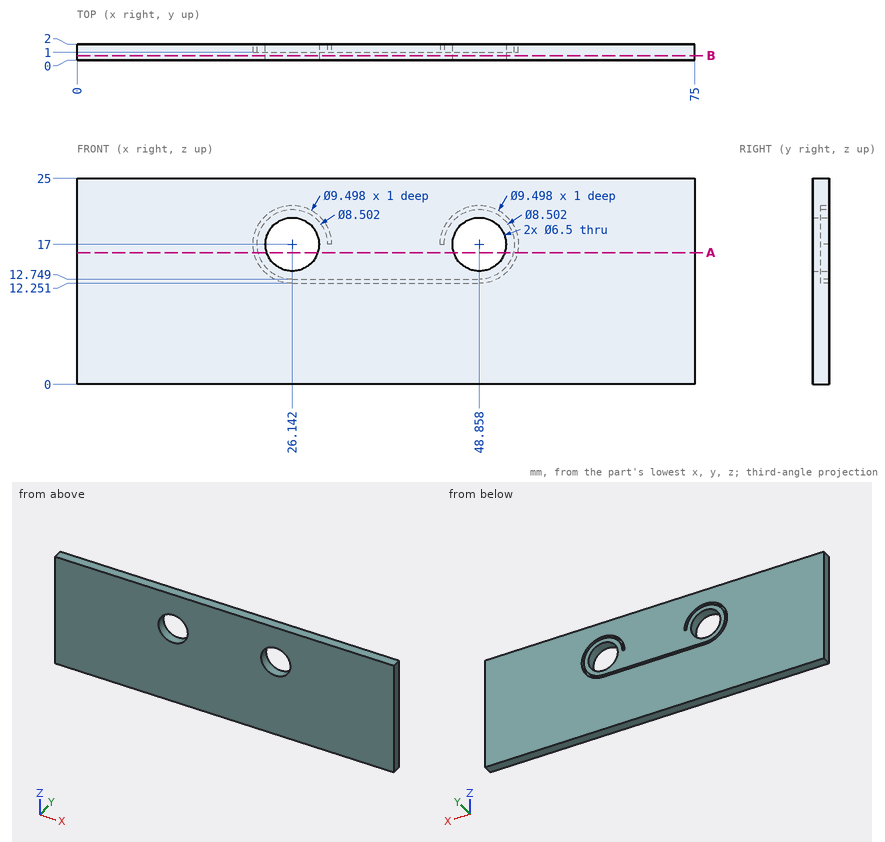
The drawing under review shows one solid part. Ordinate dimensions are in mm from its lowest x, y, z. Coordinates: 2 decimals unless noted, no trailing zeros. Loops run counter-clockwise (first coordinate to the right, second up) from the corner with the lowest first, then second, coordinate; pieces in that order, holes last. Notation, with made-up numbers: (86.25, 47) - (126.25, 47) arc R5 cw to (126.25, 55) - close; hole circle Ø7 at (76.25, 78). An arc over 180 degrees is marked (long way). Use CSV: the item, a comma, the result in double quotes. Start each with the question number.
1. Add section A-A on z = 16. Give the boundary of the cut face in (x, y), plus the area to 3 significant figures.
2. To check wall thickness, follow probe 1 along X at (y, z) = (0.5, 17); probe 2 along Z at (x, y) = (48, 1.3) (1 decimal); probe 3 along Z at (x, y) = (39, 1.65). State the ranges of each line that lie inside material, in increasing order.
3. Clearance check with a flat-ended pin moving along its axis: pin 1 (8.5 mm diameter, centred on x = 48.86, z = 17, fed in from +Y). State where the tip first meets the part, or that it passes through.
4. Add section B-B on y = 0.6. Give the boundary of the cut face in (x, z), plus the area to 3 significant figures.
Resolved:
1,outline,"(0, 0) - (23.05, 0) - (23.05, 2) - (22.01, 2) - (22.01, 1) - (21.5, 1) - (21.5, 2) - (0, 2) - close; (29.23, 0) - (45.77, 0) - (45.77, 2) - (29.23, 2) - close; (51.95, 0) - (75, 0) - (75, 2) - (53.5, 2) - (53.5, 1) - (52.99, 1) - (52.99, 2) - (51.95, 2) - close"
1,area,"124 mm2"
2,probe 1,"0 to 22.89, 29.39 to 45.61, 52.11 to 75"
2,probe 2,"0 to 12.3, 12.7 to 13.9, 20.1 to 21.2, 21.7 to 25"
2,probe 3,"0 to 12.25, 12.75 to 25"
3,pin 1,"y = 2"
4,outline,"(0, 0) - (75, 0) - (75, 25) - (0, 25) - close; hole circle Ø6.5 at (26.14, 17); hole circle Ø6.5 at (48.86, 17)"
4,area,"1,810 mm2"
